```python
from build123d import *

# Parameters (mm, degrees)
CUT_EXTRUDE_1_DEPTH = 1.5
FILLET_1_R          = 0.3
CHAMFER_1_SIZE      = 1


with BuildPart() as part:
    # Эскиз1 → Повернуть1 (revolve)
    with BuildSketch(Plane.XY):
        with BuildLine():
            Line((0, 0), (0, 3.625))
            ThreePointArc((0, 3.625), (0.908821487, 4.451033224), (2.1, 4.75))
            Line((2.1, 4.75), (2.6, 4.75))
            Line((2.6, 4.75), (2.6, 2.5))
            Line((2.6, 2.5), (18.6, 2.5))
            Line((18.6, 2.5), (18.6, 0))
            Line((18.6, 0), (0, 0))
        make_face()
    revolve(axis=Axis((18.6, 0, 0), (-1, 0, 0)))

    # Эскиз2 → Вырез-Вытянуть1 (cut)
    with BuildSketch(Plane.ZY):
        Polygon((0.866025404, 1.5), (-0.866025404, 1.5), (-1.732050808, 0), (-0.866025404, -1.5), (0.866025404, -1.5), (1.732050808, 0), align=None)
    extrude(amount=-CUT_EXTRUDE_1_DEPTH, mode=Mode.SUBTRACT)

    # Скругление1
    fillet_1_edges = [part.edges().sort_by_distance(p)[0] for p in [
        (2.6, -2.5, 0),
        (2.6, -4.75, 0),
    ]]
    fillet(fillet_1_edges, radius=FILLET_1_R)

    # Фаска1
    chamfer_1_edges = [part.edges().sort_by_distance(p)[0] for p in [
        (18.6, -2.5, 0),
    ]]
    chamfer(chamfer_1_edges, length=CHAMFER_1_SIZE)


solid = part.part
```
Read the model definition and answer for the solid it produces. Units are mm, in the model's axes. A direction names the side the tool comes from. Give positions to 0.01 mm unless a question says otherwise; leave off trailing zeros. Order: outer loops, then holes, each group sorted by start corner. A loop starts at its lowest first (then second) coordinate and runs counter-clockwise, first axis right, second up.
(1) Find section A-A (x = 8.25). Give the vertices of the cut face in (y, z).
(2) Straight lines are drawn through the part: L1, parallel to Y at x = 16.5, z = -2; L2, parallel to X at y = 3.5, z = 0.75; L3, parallel to X at y = -0.25, z = -0.5. For each, find the intervals that lie inside material, in ascending order.
(3) For a pull along Z with two mould halves and no side action, classify faces 1 (the flat face through (1, -1.5, 0)), 2 (the flat face through (18.6, 0, 0)), 3 (the cylindrical face through (10.35, -0.54, 2.44)) as released by +Z, released by -Z, zero draft, split by the parting line, or undercut.
(4) Given pin 1 (3 mm diameter, centred on x = 9.5, y = -2.5, fed in from -Z); pin 2 (1.6 mm diameter, centred on x = 0.5, z = 0.5, fed in from -Y); pin 3 (3 mm diameter, centred on x = 9, z = -0.5, fed in from -Y); pin 4 (1.5 mm diameter, centred on y = 1.5, z = 2, fed in from -X), each flat-ended and moving along its own axis, determine where each tip first touches the part or whether it passes through.
(5) For faces 4 (the flat face through (0, -2, 0)), 5 (the flat face through (1.5, 0, 0)), 6 (the flat face through (2.6, 0, 3)), determine the directions among +Z, -Z, +X, -X, +Y, -Y from which every point of the face is accessible in a straight line to the end or side of a thin tool.
Result sheet:
1. outline: circle Ø5 at (0, 0)
2. L1: y = -1.5 to 1.5
2. L2: x = 0 to 2.6
2. L3: x = 1.5 to 18.6
3. face 1: undercut
3. face 2: zero draft
3. face 3: split by the parting line
4. pin 1: stops at z = -2.29
4. pin 2: stops at y = -4.6
4. pin 3: stops at y = -2.5
4. pin 4: stops at x = 0
5. face 4: +Z, -Z, -X, +Y, -Y
5. face 5: -X
5. face 6: +X
